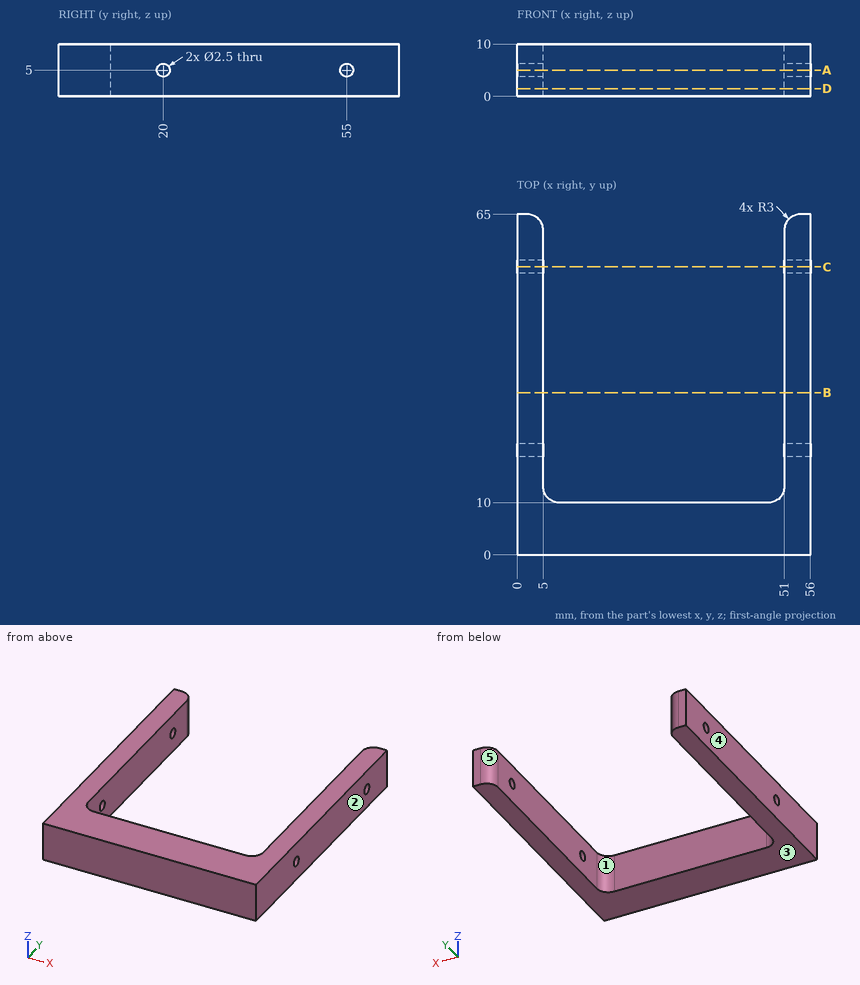
Job drawing, mm, ordinate dimensions from the low corner. One solid piece. A direction names the side the tool comes from. Coordinates: 2 decimals unless noted, no trailing zeros. Write each loop counter-clockwise with the first axis right and the second up, starting at its lowest first coordinate (ties: lowest second). Pieces come first, ordered by that corner, then holes. Notation, with made-up numbers: (48.5, 3) - (93.5, 3) arc R13 ccw to (93.5, 10) - close; hole circle Ø7 at (0, -31.5). An arc over 180 degrees is marked (long way). Use a Markdown table: item, result. Add a question column.
Item 1: Band-saw the part on D-D, the plane z = 1.5. Give the cut face in (x, y), and give its area (3 significant figures).
Item 2: Drill centre lines: L1, parallel to Y at x = 54.4, z = 5; L2, parallel to X at y = 52, z = 4.25; L3, parallel to Y at x = 52.65, z = 5. Where is each one in solid material? Low to high. Write a range as from..to.
Item 3: Band-saw the part on B-B, the plane y = 31. Give the cut face in (x, z), and give its area (3 significant figures).
Item 4: Band-saw the part on A-A, the plane z = 5. Give the cut face in (x, y), and give its area (3 significant figures).
Item 5: Mould opens along X. For the marked faces 3, 4 and 5 say: pulls with the +X half, pulls with the -X half, needs draft (parallel to the pull), parting line crosses it, or undercut.
Item 6: 3-axis set-ups, long thin cutter, end or side, ignore diameter. For the marked faces 1 and 2: which of +Z, -Z, +X, -X, +Y, -Y reach the whole face in a straight line?
Item 7: Band-saw the part on C-C, the plane y = 55. Give the cut face in (x, z), and give its area (3 significant figures).
Item 8: Flat gauge pins, fed straight in: pin 1 (4 mm diameter, centred on y = 55, z = 5, fed in from +X); pin 2 (4 mm diameter, centred on x = 28.5, z = 1, fed in from +Y). Where does each tip first touch, or does it go through?
Numbers:
| question | item | result |
|---|---|---|
| 1 | outline | (0, 0) - (56, 0) - (56, 65) - (54, 65) arc R3 ccw to (51, 62) - (51, 13) arc R3 cw to (48, 10) - (8, 10) arc R3 cw to (5, 13) - (5, 62) arc R3 ccw to (2, 65) - (0, 65) - close |
| 1 | area | 1,110 mm2 |
| 2 | L1 | 0..18.75, 21.25..53.75, 56.25..65 |
| 2 | L2 | 0..5, 51..56 |
| 2 | L3 | 0..18.75, 21.25..53.75, 56.25..64.68 |
| 3 | outline | (0, 0) - (5, 0) - (5, 10) - (0, 10) - close; (51, 0) - (56, 0) - (56, 10) - (51, 10) - close |
| 3 | area | 100 mm2 |
| 4 | outline | (0, 0) - (56, 0) - (56, 18.75) - (51, 18.75) - (51, 13) arc R3 cw to (48, 10) - (8, 10) arc R3 cw to (5, 13) - (5, 18.75) - (0, 18.75) - close; (0, 21.25) - (5, 21.25) - (5, 53.75) - (0, 53.75) - close; (0, 56.25) - (5, 56.25) - (5, 62) arc R3 ccw to (2, 65) - (0, 65) - close; (51, 21.25) - (56, 21.25) - (56, 53.75) - (51, 53.75) - close; (51, 56.25) - (56, 56.25) - (56, 65) - (54, 65) arc R3 ccw to (51, 62) - close |
| 4 | area | 1,060 mm2 |
| 5 | face 3 | needs draft |
| 5 | face 4 | pulls with the -X half |
| 5 | face 5 | undercut |
| 6 | face 1 | +Z, -Z, +Y |
| 6 | face 2 | +Z, -Z, +X, +Y, -Y |
| 7 | outline | (0, 0) - (5, 0) - (5, 3.75) - (0, 3.75) - close; (0, 6.25) - (5, 6.25) - (5, 10) - (0, 10) - close; (51, 0) - (56, 0) - (56, 3.75) - (51, 3.75) - close; (51, 6.25) - (56, 6.25) - (56, 10) - (51, 10) - close |
| 7 | area | 75.0 mm2 |
| 8 | pin 1 | x = 56 |
| 8 | pin 2 | y = 10 |
